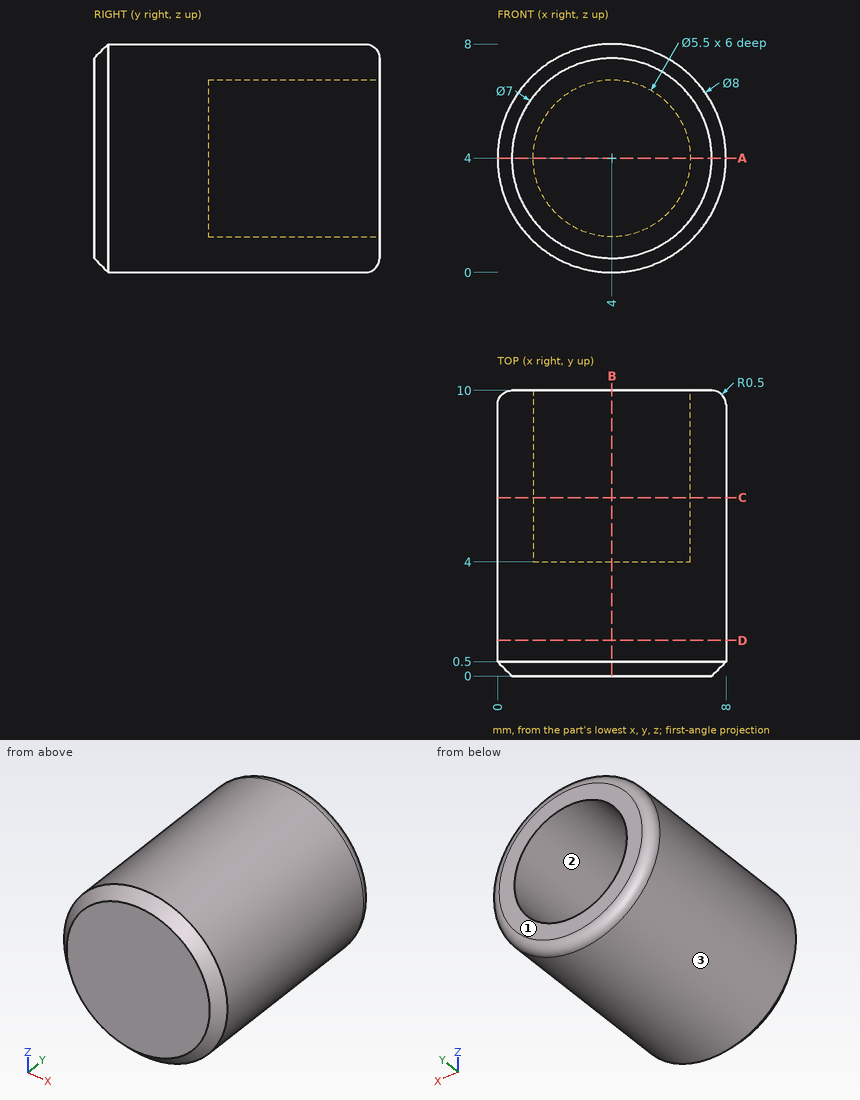
Check sheet for the drawn part. Datum: minimum x, y, z corner. Units: mm. Coordinates: 2 decimals unless noted, no trailing zeros. Order: outer loops, then holes, each group sorted by start corner. A loop starts at its lowest first (then second) coordinate and runs counter-clockwise, first axis right, second up. Notation, with made-up numbers: M 26.25,68 L 70.25,68 A15 cw 70.25,88 Z; hole C -37,76.25 d6. An arc over 180 degrees is marked long. One line per question, with ' | ' between items. Start each with the question number.
Item 1: Gauge pin test, flat ends, axial feed: P1, Ø1, axis at y = 6, z = 1.5, coming from the -X side; P2, Ø2, axis at y = 5, z = 4.5, coming from the -X side; P3, Ø3, axis at x = 6, y = 6.5, coming from the +Z side; P4, Ø2, axis at y = 4.5, z = 2.5, coming from the +X side. Record the tip position at first contact, or that the pin passes through.
Item 2: Sectioned sample at D-D on y = 1.25. Record the cut outline in (x, z).
Item 3: Sectioned sample at A-A on z = 4. Record the cut outline in (x, y).
Item 4: Material ranges on line 1 (Z direction, x = 4, y = 7.5); line 2 (Y direction, x = 5.25, z = 5.25); line 3 (X direction, y = 6, z = 6.5), recorded low to high.
Item 5: Sectioned sample at C-C on y = 6.25. Record the cut outline in (x, z), and give its area (3 significant figures).
Item 6: Mould release check, pull along X, two halves, no side actions. Record for the marked faces 1, 2 and 3: pulls with the +X half, pulls with the -X half, needs draft (parallel to the pull), parting line crosses it, or undercut.
Item 7: Sectioned sample at B-B on x = 4. Record the cut outline in (y, z), and give its area (3 significant figures).
Answer below:
1) P1: stops at x = 0.54 | P2: stops at x = 0 | P3: stops at z = 7.97 | P4: stops at x = 7.97
2) outline: C 4,4 d8
3) outline: M 0,0.5 L 0.5,0 L 7.5,0 L 8,0.5 L 8,9.5 A0.5 ccw 7.5,10 L 6.75,10 L 6.75,4 L 1.25,4 L 1.25,10 L 0.5,10 A0.5 ccw 0,9.5 Z
4) line 1: z = 0 to 1.25, 6.75 to 8 | line 2: y = 0 to 4 | line 3: x = 0.88 to 2.85, 5.15 to 7.12
5) outline: C 4,4 d8; hole C 4,4 d5.5 | area: 26.5 mm^2
6) face 1: needs draft | face 2: undercut | face 3: parting line crosses it
7) outline: M 0,0.5 L 0.5,0 L 9.5,0 A0.5 ccw 10,0.5 L 10,1.25 L 4,1.25 L 4,6.75 L 10,6.75 L 10,7.5 A0.5 ccw 9.5,8 L 0.5,8 L 0,7.5 Z | area: 46.6 mm^2
